Source: CAD feature listing. Evaluate the final solid. Frame: model axes, mm. Face numbers are marked on the shaded views. A direction names the side the tool comes from. Round coordinates to 2 decimals unless told otherwise and drop trailing zeros. Order: outer loops, then holes, each group sorted by start corner. A loop starts at its lowest first (then second) coordinate and runs counter-clockwise, first axis right, second up. Notation, with made-up numbers: (85, 9) - (129, 9) arc R10 ccw to (129, 18) - close; hole circle Ø2 at (59.25, 49.5). An arc over 180 degrees is marked (long way). Use one line per item in the form item = value. Start each with the question number.
Q1. Cut plane B-B, the plane z = 7. Return the cut outline in (x, y).
Q2. Cut plane D-D, the plane y = 11.75. Give the number of separate pieces and of enclosed holes in the cut face, and give its area (3 significant figures).
Q3. Set-up query: the marked faces 5 and 6. Return all of +Z, -Z, +X, -X, +Y, -Y with unobstructed straight access to the full face (end or side cutting, diameter ignored); none if empty.
Q4. Cut plane A-A, the plane y = 4.5. Return the cut outline in (x, z).
Q5. Ray query, line 1 (Z direction, x = 25.5, y = 23); line 2 (Z direction, x = 0, y = 1.6); line 3 (Z direction, x = 25, y = 1.05). Return the intervals inside material, ascending. Write a range as [from, to].
Q6. Pin query (flat end, axial travel): pin 1 Ø5 at (x, y) = (0, 21) entering from +Z; pin 2 Ø6.5 at (x, y) = (0, 14) entering from +Z; pin 3 Ø5 at (x, z) = (-25, 7) entering from +Y. Return the tip coordinate at first contact, or that it passes through.
Q7. Draft query along Z for the marked faces 1, 2, 3 and 4. Return one class per face: released by +Z, released by -Z, zero draft, split by the parting line, or undercut.
Q8. Cut plane C-C, the plane x = -22. Return the cut outline in (y, z).
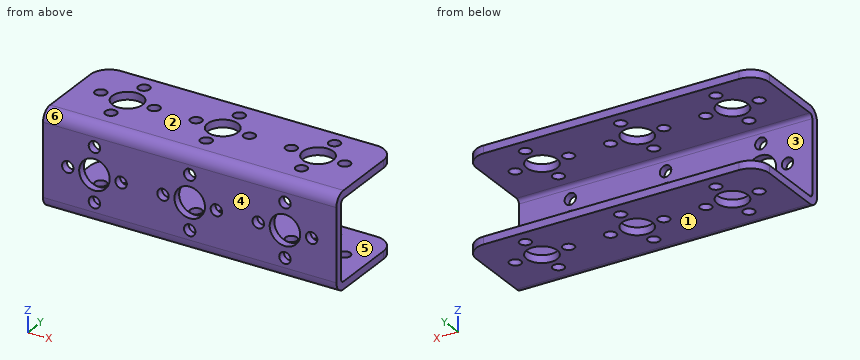
from build123d import *

# Parameters (mm, degrees)
T_LE_DE_BASE_PLI_E1_DEPTH              = 38.5
ESQUISSE7_W                            = 4
ESQUISSE7_H                            = 12.501
ESQUISSE12_W                           = 1.5
ESQUISSE12_H                           = 12.501
DIAM_TRE_DU_PER_AGE_3_0_3_1_AT_2_COUNT = 2
DIAM_TRE_DU_PER_AGE_3_0_3_1_AT_2_PITCH = 9.899494937
DIAM_TRE_DU_PER_AGE_3_0_3_1_AT_3_COUNT = 2
DIAM_TRE_DU_PER_AGE_3_0_3_1_AT_3_PITCH = 14
DIAM_TRE_DU_PER_AGE_3_0_3_1_AT_4_COUNT = 2
DIAM_TRE_DU_PER_AGE_3_0_3_1_AT_4_PITCH = 9.899494937
R_P_TITION_START                       = 10.5
R_P_TITION_CIRCULAIRE1_OUTLINE_R       = 4
R_P_TITION_CIRCULAIRE1_OUTLINE_R_2     = 1.5
R_P_TITION_CIRCULAIRE1_DEPTH           = 2
R_P_TITION_CIRCULAIRE1_2_OUTLINE_R     = 4
R_P_TITION_CIRCULAIRE1_2_OUTLINE_R_2   = 1.5
R_P_TITION_CIRCULAIRE1_2_DEPTH         = 2
R_P_TITION_LIN_AIRE1_COUNT             = 3
R_P_TITION_LIN_AIRE1_PITCH             = 25
R_P_TITION_LIN_AIRE1_COPY_1_SKETCH_W   = 1.5
R_P_TITION_LIN_AIRE1_COPY_1_SKETCH_H   = 12.501
R_P_TITION_LIN_AIRE1_COPY_2_SKETCH_W   = 1.5
R_P_TITION_LIN_AIRE1_COPY_2_SKETCH_H   = 12.501
R_P_TITION_LIN_AIRE1_COPY_3_SKETCH_W   = 1.5
R_P_TITION_LIN_AIRE1_COPY_3_SKETCH_H   = 12.501
R_P_TITION_LIN_AIRE1_COPY_4_SKETCH_W   = 1.5
R_P_TITION_LIN_AIRE1_COPY_4_SKETCH_H   = 12.501
R_P_TITION_LIN_AIRE1_COPY_5_SKETCH_W   = 1.5
R_P_TITION_LIN_AIRE1_COPY_5_SKETCH_H   = 12.501
R_P_TITION_LIN_AIRE1_COPY_6_SKETCH_W   = 1.5
R_P_TITION_LIN_AIRE1_COPY_6_SKETCH_H   = 12.501
CONG_1_R                               = 5


# Read off the part's stored shape, not the designer's step: Répétition circulaire1
# Sheet-metal steps are written as plain solids
with BuildPart() as part:
    # Esquisse1 → Tôle de base pliée1 (new, symmetric)
    with BuildSketch(Plane(origin=(0, 0, 0), x_dir=(0, 0, -1), z_dir=(1, 0, 0))):
        with BuildLine():
            Line((-12.5, 25), (-12.5, 3))
            ThreePointArc((-12.5, 3), (-11.621320344, 0.878679656), (-9.5, 0))
            Line((-9.5, 0), (9.5, 0))
            ThreePointArc((9.5, 0), (11.621320344, 0.878679656), (12.5, 3))
            Line((12.5, 3), (12.5, 25))
            Line((12.5, 25), (10.5, 25))
            Line((10.5, 25), (10.5, 3))
            ThreePointArc((10.5, 3), (10.207106781, 2.292893219), (9.5, 2))
            Line((9.5, 2), (-9.5, 2))
            ThreePointArc((-9.5, 2), (-10.207106781, 2.292893219), (-10.5, 3))
            Line((-10.5, 3), (-10.5, 25))
            Line((-10.5, 25), (-12.5, 25))
        make_face()
    extrude(amount=T_LE_DE_BASE_PLI_E1_DEPTH, both=True)

    # Esquisse7 → Diamètre du perçage Ø8.0 (8)1 (revolve, cut)
    with BuildSketch(Plane(origin=(25, 14, 0), x_dir=(0, -1, 0), z_dir=(1, 0, 0))):
        with Locations((2, 6.2505)):
            Rectangle(ESQUISSE7_W, ESQUISSE7_H)
    diam_tre_du_per_age_8_0_8_1 = revolve(axis=Axis((25, 14, 6.35), (0, 0, -1)), mode=Mode.SUBTRACT)

    # Esquisse12 → Diamètre du perçage Ø3.0 (3)1 (revolve, cut)
    with BuildSketch(Plane(origin=(25, 21, 0), x_dir=(0, -1, 0), z_dir=(1, 0, 0))):
        with Locations((0.75, 6.2505)):
            Rectangle(ESQUISSE12_W, ESQUISSE12_H)
    diam_tre_du_per_age_3_0_3_1 = revolve(axis=Axis((25, 21, 6.35), (0, 0, -1)), mode=Mode.SUBTRACT)

    # Diamètre du perçage Ø3.0 (3)1 at 2: Diamètre du perçage Ø3.0 (3)1 ×2
    with Locations(*[Vector(-0.7071067811865475, -0.7071067811865478, 0) * (i * DIAM_TRE_DU_PER_AGE_3_0_3_1_AT_2_PITCH) for i in range(1, DIAM_TRE_DU_PER_AGE_3_0_3_1_AT_2_COUNT)]):
        add(diam_tre_du_per_age_3_0_3_1, mode=Mode.SUBTRACT)

    # Diamètre du perçage Ø3.0 (3)1 at 3: Diamètre du perçage Ø3.0 (3)1 ×2
    with Locations(*[(0, -i * DIAM_TRE_DU_PER_AGE_3_0_3_1_AT_3_PITCH, 0) for i in range(1, DIAM_TRE_DU_PER_AGE_3_0_3_1_AT_3_COUNT)]):
        add(diam_tre_du_per_age_3_0_3_1, mode=Mode.SUBTRACT)

    # Diamètre du perçage Ø3.0 (3)1 at 4: Diamètre du perçage Ø3.0 (3)1 ×2
    with Locations(*[Vector(0.7071067811865476, -0.7071067811865476, 0) * (i * DIAM_TRE_DU_PER_AGE_3_0_3_1_AT_4_PITCH) for i in range(1, DIAM_TRE_DU_PER_AGE_3_0_3_1_AT_4_COUNT)]):
        add(diam_tre_du_per_age_3_0_3_1, mode=Mode.SUBTRACT)

    # Répétition circulaire1 outline → Répétition circulaire1 (cut)
    with BuildSketch(Plane.XY.offset(R_P_TITION_START)):
        with Locations((25, 14)):
            Circle(R_P_TITION_CIRCULAIRE1_OUTLINE_R)
        with Locations((32, 14)):
            Circle(R_P_TITION_CIRCULAIRE1_OUTLINE_R_2)
        with Locations((25, 7)):
            Circle(R_P_TITION_CIRCULAIRE1_OUTLINE_R_2)
        with Locations((18, 14)):
            Circle(R_P_TITION_CIRCULAIRE1_OUTLINE_R_2)
        with Locations((25, 21)):
            Circle(R_P_TITION_CIRCULAIRE1_OUTLINE_R_2)
    r_p_tition_circulaire1 = extrude(amount=R_P_TITION_CIRCULAIRE1_DEPTH, mode=Mode.SUBTRACT)

    # R_p_tition circulaire1 2 outline → R_p_tition circulaire1 2 (cut)
    with BuildSketch(Plane(origin=(0, 0, 0), x_dir=(1, 0, 0), z_dir=(0, 1, 0))):
        with Locations((25, 0)):
            Circle(R_P_TITION_CIRCULAIRE1_2_OUTLINE_R)
        with Locations((32, 0)):
            Circle(R_P_TITION_CIRCULAIRE1_2_OUTLINE_R_2)
        with Locations((25, -7)):
            Circle(R_P_TITION_CIRCULAIRE1_2_OUTLINE_R_2)
        with Locations((18, 0)):
            Circle(R_P_TITION_CIRCULAIRE1_2_OUTLINE_R_2)
        with Locations((25, 7)):
            Circle(R_P_TITION_CIRCULAIRE1_2_OUTLINE_R_2)
    r_p_tition_circulaire1_2 = extrude(amount=R_P_TITION_CIRCULAIRE1_2_DEPTH, mode=Mode.SUBTRACT)

    # Répétition linéaire1: Diamètre du perçage Ø8.0 (8)1, Diamètre du perçage Ø3.0 (3)1, Répétition circulaire1, R_p_tition circulaire1 2 ×3
    with Locations(*[(-i * R_P_TITION_LIN_AIRE1_PITCH, 0, 0) for i in range(1, R_P_TITION_LIN_AIRE1_COUNT)]):
        add(diam_tre_du_per_age_8_0_8_1, mode=Mode.SUBTRACT)
        add(diam_tre_du_per_age_3_0_3_1, mode=Mode.SUBTRACT)
        add(r_p_tition_circulaire1, mode=Mode.SUBTRACT)
        add(r_p_tition_circulaire1_2, mode=Mode.SUBTRACT)

    # Répétition linéaire1 copy 1 sketch → Répétition linéaire1 copy 1 (revolve, cut)
    with BuildSketch(Plane(origin=(-7, 14, 0), x_dir=(0, -1, 0), z_dir=(1, 0, 0))):
        with Locations((0.75, 6.2505)):
            Rectangle(R_P_TITION_LIN_AIRE1_COPY_1_SKETCH_W, R_P_TITION_LIN_AIRE1_COPY_1_SKETCH_H)
    revolve(axis=Axis((-7, 14, 6.35), (0, 0, -1)), mode=Mode.SUBTRACT)

    # Répétition linéaire1 copy 2 sketch → Répétition linéaire1 copy 2 (revolve, cut)
    with BuildSketch(Plane(origin=(-32, 14, 0), x_dir=(0, -1, 0), z_dir=(1, 0, 0))):
        with Locations((0.75, 6.2505)):
            Rectangle(R_P_TITION_LIN_AIRE1_COPY_2_SKETCH_W, R_P_TITION_LIN_AIRE1_COPY_2_SKETCH_H)
    revolve(axis=Axis((-32, 14, 6.35), (0, 0, -1)), mode=Mode.SUBTRACT)

    # Répétition linéaire1 copy 3 sketch → Répétition linéaire1 copy 3 (revolve, cut)
    with BuildSketch(Plane(origin=(0, 7, 0), x_dir=(0, -1, 0), z_dir=(1, 0, 0))):
        with Locations((0.75, 6.2505)):
            Rectangle(R_P_TITION_LIN_AIRE1_COPY_3_SKETCH_W, R_P_TITION_LIN_AIRE1_COPY_3_SKETCH_H)
    revolve(axis=Axis((0, 7, 6.35), (0, 0, -1)), mode=Mode.SUBTRACT)

    # Répétition linéaire1 copy 4 sketch → Répétition linéaire1 copy 4 (revolve, cut)
    with BuildSketch(Plane(origin=(-25, 7, 0), x_dir=(0, -1, 0), z_dir=(1, 0, 0))):
        with Locations((0.75, 6.2505)):
            Rectangle(R_P_TITION_LIN_AIRE1_COPY_4_SKETCH_W, R_P_TITION_LIN_AIRE1_COPY_4_SKETCH_H)
    revolve(axis=Axis((-25, 7, 6.35), (0, 0, -1)), mode=Mode.SUBTRACT)

    # Répétition linéaire1 copy 5 sketch → Répétition linéaire1 copy 5 (revolve, cut)
    with BuildSketch(Plane(origin=(7, 14, 0), x_dir=(0, -1, 0), z_dir=(1, 0, 0))):
        with Locations((0.75, 6.2505)):
            Rectangle(R_P_TITION_LIN_AIRE1_COPY_5_SKETCH_W, R_P_TITION_LIN_AIRE1_COPY_5_SKETCH_H)
    revolve(axis=Axis((7, 14, 6.35), (0, 0, -1)), mode=Mode.SUBTRACT)

    # Répétition linéaire1 copy 6 sketch → Répétition linéaire1 copy 6 (revolve, cut)
    with BuildSketch(Plane(origin=(-18, 14, 0), x_dir=(0, -1, 0), z_dir=(1, 0, 0))):
        with Locations((0.75, 6.2505)):
            Rectangle(R_P_TITION_LIN_AIRE1_COPY_6_SKETCH_W, R_P_TITION_LIN_AIRE1_COPY_6_SKETCH_H)
    revolve(axis=Axis((-18, 14, 6.35), (0, 0, -1)), mode=Mode.SUBTRACT)

    # Congé1
    cong_1_edges = [part.edges().sort_by_distance(p)[0] for p in [
        (-38.5, 25, 11.5),
        (-38.5, 25, -11.5),
        (38.5, 25, 11.5),
        (38.5, 25, -11.5),
    ]]
    fillet(cong_1_edges, radius=CONG_1_R)


solid = part.part
Completed:
q1.outline = (-38.5, 0) - (-26.5, 0) - (-26.5, 2) - (-38.5, 2) - close; (-23.5, 0) - (-1.5, 0) - (-1.5, 2) - (-23.5, 2) - close; (1.5, 0) - (23.5, 0) - (23.5, 2) - (1.5, 2) - close; (26.5, 0) - (38.5, 0) - (38.5, 2) - (26.5, 2) - close
q2.separate_pieces = 8
q2.enclosed_holes = 0
q2.area = 229 mm2
q3.face_5 = +X, -X, +Y
q3.face_6 = +Z, +X, -X, -Y
q4.outline = (-38.5, -12.5) - (38.5, -12.5) - (38.5, -10.5) - (-38.5, -10.5) - close; (-38.5, 10.5) - (38.5, 10.5) - (38.5, 12.5) - (-38.5, 12.5) - close
q5.line_1 = [-12.5, -10.5], [10.5, 12.5]
q5.line_2 = [-12.15, -8.5], [-5.5, -4], [4, 5.5], [8.5, 12.15]
q5.line_3 = [-11.78, -8.5], [-5.5, -4], [4, 5.5], [8.5, 11.78]
q6.pin_1 = 12.5
q6.pin_2 = through
q6.pin_3 = 2
q7.face_1 = released by -Z
q7.face_2 = released by +Z
q7.face_3 = undercut
q7.face_4 = zero draft
q8.outline = (0, -9.5) arc R3 ccw to (3, -12.5) - (11.35, -12.5) - (11.35, -10.5) - (3, -10.5) arc R1 cw to (2, -9.5) - (2, -2.65) - (0, -2.65) - close; (0, 2.65) - (2, 2.65) - (2, 9.5) arc R1 cw to (3, 10.5) - (11.35, 10.5) - (11.35, 12.5) - (3, 12.5) arc R3 ccw to (0, 9.5) - close; (16.65, -12.5) - (25, -12.5) - (25, -10.5) - (16.65, -10.5) - close; (16.65, 10.5) - (25, 10.5) - (25, 12.5) - (16.65, 12.5) - close
